Can you work these out from the model? Positions are in its coordinate system, mm. Face numbers are marked on the shaded views. Coordinates: 2 decimals unless noted, no trailing zeros. Loops run counter-clockwise (first coordinate to the right, second up) from the corner with the lowest first, then second, coordinate; pieces in that order, holes last. Notation, with made-up numbers: M 51.5,-24.5 L 105.5,-24.5 A26 cw 105.5,0.5 Z; hole C -29,4 d1. An arc over 180 degrees is marked long. Answer as a JSON object with one key per item and string values. Group by question number.
Item 1: I'm going to push flat-ended pins straight in: pin 1 Ø4 at (x, y) = (-55, -9) entering from -Z; pin 2 Ø1.3 at (y, z) = (15.5, 0) entering from +X; pin 3 Ø12 at (y, z) = (-4, -7.5) entering from -X. Where does each tip first touch, or does it pass through?
Item 2: Suppose I cut it at B-B (x = 26). Write out the boundary of the cut face in (y, z), then the cut area to 3 significant figures.
Item 3: If I drill on line 1 (Z direction, x = 39, y = 0); line 2 (Z direction, x = -49, y = 0), over which ranges is the centre line in solid material (lowest first)?
Item 4: We'd pull the mould along Z, two halves only. Please class the marked faces 1, 2 and 3: +Z half, -Z half, draft (parallel to the pull), parting line (faces both ways), or undercut.
Item 5: Suppose I cut it at A-A (x = -80). Write out the boundary of the cut face in (y, z).
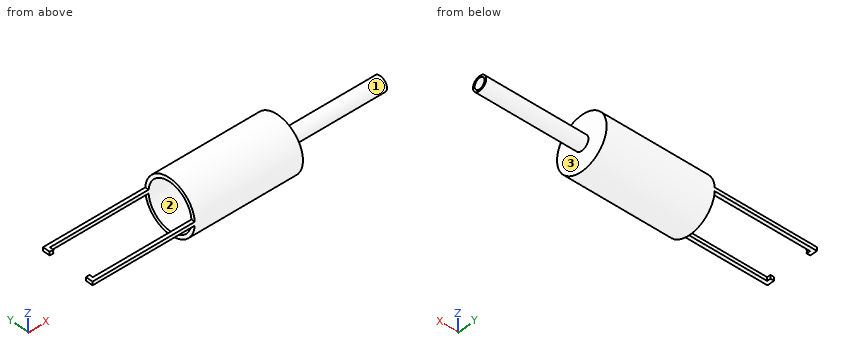
```python
from build123d import *

# Parameters (mm, degrees)
F0_R     = 19.05
F1_DEPTH = 148.2
F4_W     = 101.6
F4_H     = 31.79568
F5_DEPTH = 25.4
F6_R     = 5.08
F7_DEPTH = 72
F8_R     = 3.81
F9_DEPTH = 152.4


with BuildPart() as f1:
    # F0 (on Right) → F1 (new body)
    with BuildSketch(Plane.YZ):
        Circle(F0_R)
    extrude(amount=-F1_DEPTH)

    # F2 (on Front) → F3 (revolve, cut)
    with BuildSketch(Plane.XZ):
        with BuildLine():
            ThreePointArc((-8.89, -16.51), (-4.182231, -8.844527), (-2.54, 0))
            Line((-2.54, 0), (-8.89, 0))
            Line((-8.89, 0), (-8.89, -16.51))
        make_face()
        Polygon((-8.89, -16.51), (-8.89, 0), (-148.2, 0), (-148.2, -13.97), (-145.66, -13.97), (-145.66, -16.51), (-76.2, -16.51), align=None)
    revolve(axis=Axis((-78.545, 0, 0), (-1, 0, 0)), mode=Mode.SUBTRACT)

    # F4 (on Front) → F5 (cut, symmetric)
    with BuildSketch(Plane.XZ):
        Polygon((-177.8, 1.27), (-76.2, 1.27), (-76.2, 26.052563), (-178.992286, 26.052563), align=None)
        with Locations((-127, -17.16784)):
            Rectangle(F4_W, F4_H)
    extrude(amount=F5_DEPTH, both=True, mode=Mode.SUBTRACT)

    # F6 (on face) → F7 (join)
    with BuildSketch(Plane.YZ):
        Circle(F6_R)
    extrude(amount=F7_DEPTH)

    # F8 (on face) → F9 (cut)
    with BuildSketch(Plane.YZ.offset(72)):
        Circle(F8_R)
    extrude(amount=-F9_DEPTH, mode=Mode.SUBTRACT)


solid = f1.part
```
From the geometry:
{
 "1": {"pin 1": "z = -17.72", "pin 2": "x = 0", "pin 3": "x = -7.26"},
 "2": {"outline": "C 0,0 d10.16; hole C 0,0 d7.62", "area": "35.5 mm2"},
 "3": {"line 1": "-5.08 to -3.81, 3.81 to 5.08", "line 2": "-19.05 to -16.51, 16.51 to 19.05"},
 "4": {"face 1": "parting line", "face 2": "undercut", "face 3": "draft"},
 "5": {"outline": "M -19.01,-1.27 L -16.46,-1.27 A16.51 cw -16.46,1.27 L -19.01,1.27 A19.05 ccw Z; M 16.46,-1.27 L 19.01,-1.27 A19.05 ccw 19.01,1.27 L 16.46,1.27 A16.51 cw Z"}
}
